Work out the finished part from the listing and answer in its coordinate system (mm). A direction names the side the tool comes from. Give positions to 0.01 mm unless a question says otherwise; leave off trailing zeros. Write each loop counter-clockwise with the first axis right and the second up, starting at its lowest first coordinate (ties: lowest second). Pieces come first, ordered by that corner, then holes. Notation, with made-up numbers: (13, 40) -> (29, 40) arc R27 ccw to (29, 68) -> close; hole circle Ø10 at (-1.75, 28). An arc over 180 degrees is marked (long way). Use a Markdown table: item, result. Add a question column.
Q1. For a pull along Z with two mould halves and no side action, classify faces 1 (the face through (6, 1.588, -64)), 2 (the face through (8.66, 1, -32)), 3 (the face through (6, 1, -101.538)) as pulls with the +Z half, pulls with the -Z half, needs draft (parallel to the pull), parting line crosses it, or undercut.
Q2. Consider line 1 (Z direction, x = 5.75, y = 0.2); line 2 (X direction, y = 1.2, z = -95.5). Determine where each line is inside the solid, lowest interval first.
Q3. Section B-B, the plane x = 6.5 is taken. Give the vertices of the cut face in (y, z).
Q4. Section A-A, the plane y = 1 is taken. Give the vertices of the cut face in (x, z), plus the area to 3 significant figures.
Q5. For faces 4 (the face through (0, 1, -63)), 5 (the face through (6, 1, -92.875)), determine the directions among +Z, -Z, +X, -X, +Y, -Y from which every point of the face is accessible in a straight line to the end or side of a thin tool.
from build123d import *

# Parameters (mm, degrees)
SKETCH1_W           = 12.7
SKETCH1_H           = 76.2
SKETCH1_W_2         = 4.6228
SKETCH1_H_2         = 4.6228
SKETCH1_W_3         = 4.62
BOSS_EXTRUDE1_DEPTH = 1.5875


with BuildPart() as part:
    # Sketch1 → Boss-Extrude1 (new body)
    with BuildSketch(Plane(origin=(0, 0, 0), x_dir=(1, 0, 0), z_dir=(0, 1, 0))):
        with Locations((6.35, 63.437542426)):
            Rectangle(SKETCH1_W, SKETCH1_H)
        with Locations((6.3486, 95.186142426)):
            Rectangle(SKETCH1_W_2, SKETCH1_H_2, mode=Mode.SUBTRACT)
        with Locations((6.35, 31.688942426)):
            Rectangle(SKETCH1_W_3, SKETCH1_H_2, mode=Mode.SUBTRACT)
    extrude(amount=BOSS_EXTRUDE1_DEPTH)


solid = part.part
Result set:
| question | item | result |
|---|---|---|
| 1 | face 1 | needs draft |
| 1 | face 2 | undercut |
| 1 | face 3 | pulls with the -Z half |
| 2 | line 1 | z = -101.54 to -97.5, -92.87 to -34, -29.38 to -25.34 |
| 2 | line 2 | x = 0 to 4.04, 8.66 to 12.7 |
| 3 | outline | (0, -101.54) -> (1.59, -101.54) -> (1.59, -97.5) -> (0, -97.5) -> close; (0, -92.87) -> (1.59, -92.87) -> (1.59, -34) -> (0, -34) -> close; (0, -29.38) -> (1.59, -29.38) -> (1.59, -25.34) -> (0, -25.34) -> close |
| 4 | outline | (0, -101.54) -> (12.7, -101.54) -> (12.7, -25.34) -> (0, -25.34) -> close; hole (4.04, -97.5) -> (8.66, -97.5) -> (8.66, -92.87) -> (4.04, -92.87) -> close; hole (4.04, -34) -> (8.66, -34) -> (8.66, -29.38) -> (4.04, -29.38) -> close |
| 4 | area | 925 mm2 |
| 5 | face 4 | +Z, -Z, -X, +Y, -Y |
| 5 | face 5 | +Y, -Y |
